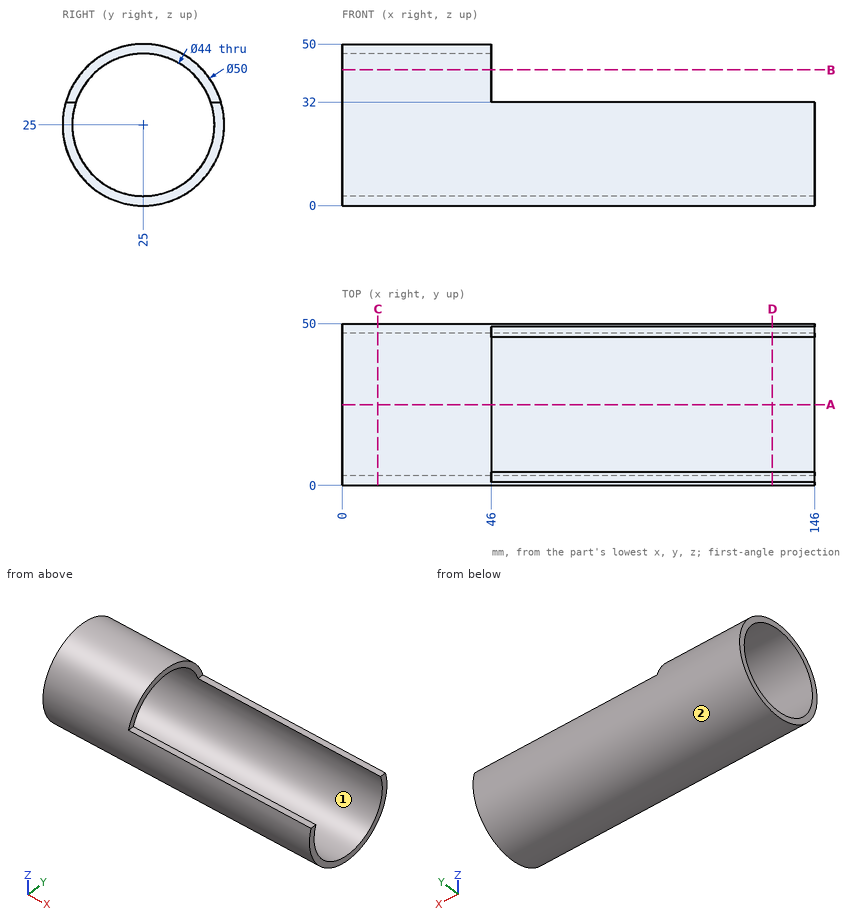
Part print with two shaded views. Sizes in mm from the minimum x, y, z corner. Coordinates: 2 decimals unless noted, no trailing zeros. Loops run counter-clockwise (first coordinate to the right, second up) from the corner with the lowest first, then second, coordinate; pieces in that order, holes last. Notation, with made-up numbers: (5.25, -34.5) - (35.25, -34.5) arc R18 cw to (35.25, -6.5) - close; hole circle Ø2 at (-35.5, -38.75). An arc over 180 degrees is marked (long way). Write each question's results on one line, items separated by ' | '. Start each with the question number.
Q1. Probe line 1 along Y through (x, z) = (116.5, 25); line 2 along Z through (x, y) = (78, 25). List the from-to ranges inside material, lowest first.
Q2. Slice it at D-D on x = 133. Give the cut face in (y, z).
Q3. Slice it at B-B on z = 42. Give the cut face in (x, y), and give its area (3 significant figures).
Q4. Two-plate mould, pull along Y, no slides. Class the marked faces 1 and 2: +Y half, -Y half, draft (parallel to the pull), parting line (faces both ways), or undercut.
Q5. Slice it at C-C on x = 11. Give the cut face in (y, z), and give its area (3 significant figures).
Q6. Drop flat-ended pins along their axis: pin 1 Ø9 at (y, z) = (13, 44.5) entering from +X; pin 2 Ø10 at (x, y) = (25.5, 36) entering from -Z; pin 3 Ø10 at (x, z) = (55.5, 12) entering from +Y. Give the stop position or say it passes through.
Q7. Slice it at A-A on y = 25. Give the cut face in (x, z).
Answer:
1) line 1: y = 0 to 3, 47 to 50 | line 2: z = 0 to 3
2) outline: (1, 32) arc R25 ccw (long way) to (49, 32) - (45.86, 32) arc R22 cw (long way) to (4.14, 32) - close
3) outline: (0, 6.67) - (46, 6.67) - (46, 11.04) - (0, 11.04) - close; (0, 38.96) - (46, 38.96) - (46, 43.33) - (0, 43.33) - close | area: 402 mm2
4) face 1: undercut | face 2: parting line
5) outline: circle Ø50 at (25, 25); hole circle Ø44 at (25, 25) | area: 443 mm2
6) pin 1: stops at x = 46 | pin 2: stops at z = 0.73 | pin 3: stops at y = 48.69
7) outline: (0, 0) - (146, 0) - (146, 3) - (0, 3) - close; (0, 47) - (46, 47) - (46, 50) - (0, 50) - close
